Geometry check sheet. Reference: the model listing, model coordinates, mm. A direction names the side the tool comes from. Coordinates: 2 decimals unless noted, no trailing zeros. Order: outer loops, then holes, each group sorted by start corner. A loop starts at its lowest first (then second) coordinate and runs counter-clockwise, first axis right, second up. Notation, with made-up numbers: (21.25, 25) - (39.25, 25) arc R19 cw to (39.25, 52) - close; hole circle Ø5 at (1.25, 15). An arc over 180 degrees is marked (long way). Use CSV: the item, a comma, the result in double quotes. Start each with the question number.
1) Draft check along Y on faces 4 (the flat face through (151, 0, 1)), 5 (the flat face through (151, -191.008, 1)), 6 (the flat face through (13, -13, 0)), 7 (the flat face through (180, -52, 3.81)). Enter one of: released by +Y, released by -Y, zero draft, split by the parting line, or undercut.
2) Thickness scan on probe 1 along X at (y, z) = (-141.5, -0.25); probe 2 along Y at (x, z) = (122.5, -1.5); probe 3 along X at (y, z) = (-56, 3.25). Record the ranges inside material, lowest first. Write a range as [from, to].
3) Tool access check on faces 1 (the flat face through (13, -178, 0)), 2 (the flat face through (185, -52, -2.54)), 3 (the flat face through (108, -77, 0)). Record the directions out of +Z, -Z, +X, -X, +Y, -Y that give a thin tool (end or side, any length) a straight path to the whole face; none if there is none.
4) Sectioned sample at A-A, the plane y = -74.5. Record the cut outline in (x, z).
5) Sectioned sample at C-C, the plane x = 146. Record the cut outline in (y, z), and give its area (3 significant figures).
6) Depth check by flat-ended pin: P1, Ø8, axis at x = 285.877, y = -178.181, coming from the +Z side. Enter the tip coordinate at first touch or a pass-through.
7) Sectioned sample at B-B, the plane z = 1.5. Record the cut outline in (x, y) (3 decimals).
from build123d import *

# Parameters (mm, degrees)
SKETCH1_W           = 298.704
SKETCH1_H           = 191.008
SKETCH1_R           = 6.477
SKETCH1_R_2         = 45.085
BOSS_EXTRUDE1_DEPTH = 3.81
SKETCH3_W           = 298.704
SKETCH3_H           = 191.008
SKETCH3_R           = 47.625
BOSS_EXTRUDE2_DEPTH = 2.54
CUT_EXTRUDE1_START  = -3.81
SKETCH4_R           = 50.165
CUT_EXTRUDE1_DEPTH  = 2.54


with BuildPart() as part:
    # Sketch1 → Boss-Extrude1 (new body)
    with BuildSketch(Plane.XY):
        with Locations((149.352, -95.504)):
            Rectangle(SKETCH1_W, SKETCH1_H)
        with Locations(Location((12.827, -12.827, 0), (0, 0, 180))):
            Circle(SKETCH1_R, mode=Mode.SUBTRACT)
        with Locations(Location((285.877, -12.827, 0), (0, 0, 180))):
            Circle(SKETCH1_R, mode=Mode.SUBTRACT)
        with Locations(Location((285.877, -178.181, 0), (0, 0, 180))):
            Circle(SKETCH1_R, mode=Mode.SUBTRACT)
        with Locations(Location((12.827, -178.181, 0), (0, 0, 180))):
            Circle(SKETCH1_R, mode=Mode.SUBTRACT)
        with Locations(Location((149.352, -95.504, 0), (0, 0, 180))):
            Circle(SKETCH1_R_2, mode=Mode.SUBTRACT)
    extrude(amount=BOSS_EXTRUDE1_DEPTH)

    # Sketch3 → Boss-Extrude2 (add)
    with BuildSketch(Plane(origin=(0, 0, 0), x_dir=(-1, 0, 0), z_dir=(0, 0, -1))):
        with Locations((-149.352, -95.504)):
            Rectangle(SKETCH3_W, SKETCH3_H)
        with Locations((-149.352, -95.504)):
            Circle(SKETCH3_R, mode=Mode.SUBTRACT)
    extrude(amount=BOSS_EXTRUDE2_DEPTH)

    # Sketch4 → Cut-Extrude1 (cut)
    with BuildSketch(Plane.XY.offset(3.81).offset(CUT_EXTRUDE1_START)):
        with Locations((149.352, -95.504)):
            Circle(SKETCH4_R)
    extrude(amount=-CUT_EXTRUDE1_DEPTH, mode=Mode.SUBTRACT)


solid = part.part
Evaluation:
1,face 4,"released by +Y"
1,face 5,"released by -Y"
1,face 6,"undercut"
1,face 7,"zero draft"
2,probe 1,"[0, 129.33], [169.37, 298.7]"
2,probe 2,"[-191.01, -137.88], [-53.13, 0]"
2,probe 3,"[0, 127.62], [171.08, 298.7]"
3,face 1,"+Z"
3,face 2,"-Z, +X, -X, +Y, -Y"
3,face 3,"-Z"
4,outline,"(0, -2.54) - (103.8, -2.54) - (103.8, 0) - (109.46, 0) - (109.46, 3.81) - (0, 3.81) - close; (189.25, 0) - (194.91, 0) - (194.91, -2.54) - (298.7, -2.54) - (298.7, 3.81) - (189.25, 3.81) - close"
5,outline,"(-191.01, -2.54) - (-145.56, -2.54) - (-145.56, 0) - (-140.46, 0) - (-140.46, 3.81) - (-191.01, 3.81) - close; (-50.54, 0) - (-45.45, 0) - (-45.45, -2.54) - (0, -2.54) - (0, 3.81) - (-50.54, 3.81) - close"
5,area,"616 mm²"
6,P1,"z = 0"
7,outline,"(0, -191.008) - (298.704, -191.008) - (298.704, 0) - (0, 0) - close; hole circle Ø12.954 at (12.827, -178.181); hole circle Ø12.954 at (12.827, -12.827); hole circle Ø90.17 at (149.352, -95.504); hole circle Ø12.954 at (285.877, -178.181); hole circle Ø12.954 at (285.877, -12.827)"
